Read the model definition and answer for the solid it produces. Units are mm, in the model's axes. A direction names the side the tool comes from. Coordinates: 2 decimals unless noted, no trailing zeros. Loops run counter-clockwise (first coordinate to the right, second up) from the corner with the lowest first, then second, coordinate; pieces in that order, holes last.
Q1. Section D-D (y = 4.55) is taken. Count the separate pieces of the cut face and the enclosed holes in it, then the cut area to 3 significant figures.
Q2. Which of the six approach directions +Z, -Z, +X, -X, +Y, -Y give full straight-line access (tool end or side, diameter ignored) to faces 1 (the face through (166, 3, -151)), 2 (the face through (166, 3, -223)), 3 (the face through (133.805, 3, -141))?
Q3. Section B-B (z = -150.5) is taken. Give the vertices of the cut face in (x, y).
Q4. Flat-ended cylindrical pins translate along their axes: P1, Ø1.8, axis at x = 119.5, y = 2, coming from the +Z side (3 decimals); P2, Ø1, axis at x = 152.5, y = 3, coming from the +Z side; P3, Ø4, axis at x = 126.5, z = -252, coming from the -Y side; P4, Ø3, axis at y = 3, z = -157, coming from the +X side. Find the tip coordinate at first contact, or state that the pin passes through.
Q5. Straight lines are drawn through the part: line 1 (X direction, y = 1.7, z = -183.5); line 2 (Z direction, x = 120, y = 1.45) (3 decimals); line 3 (X direction, y = 3.6, z = -250). For each, find the intervals that lie inside material, in ascending order.
Q6. The mould has two halves that part along X. Classify faces 4 (the face through (146, 3, -144)), 5 (the face through (146, 0, -205)), 6 (the face through (166, 3, -259)): pulls with the +X half, pulls with the -X half, needs draft (parallel to the pull), parting line crosses it, or undercut.
Q7. Section C-C (x = 136.5) is taken. Give the vertices of the cut face in (y, z).
Q8. Section A-A (x = 148.5) is taken. Give the vertices of the cut face in (y, z).
from build123d import *

# Parameters (mm, degrees)
BOSS_EXTRUDE1_DEPTH = 6
SKETCH3_W           = 20
SKETCH3_H           = 20
SKETCH3_W_2         = 5
SKETCH3_H_2         = 10
CUT_EXTRUDE1_DEPTH  = 6


with BuildPart() as part:
    # Sketch2 → Boss-Extrude1 (new body)
    with BuildSketch(Plane(origin=(0, 0, 0), x_dir=(1, 0, 0), z_dir=(0, 1, 0))):
        Polygon((121, 270), (121, 240.585), (115, 240.585), (115, 216.195), (121, 216.195), (121, 191.805), (115, 191.805), (115, 167.415), (121, 167.415), (121, 143.025), (121, 138), (133.805, 138), (133.805, 144), (158.195, 144), (158.195, 138), (171, 138), (171, 167.415), (177, 167.415), (177, 191.805), (171, 191.805), (171, 216.195), (177, 216.195), (177, 240.585), (171, 240.585), (171, 264.975), (171, 270), (158.195, 270), (158.195, 264), (133.805, 264), (133.805, 270), align=None)
    extrude(amount=BOSS_EXTRUDE1_DEPTH)

    # Sketch3 → Cut-Extrude1 (cut)
    with BuildSketch(Plane(origin=(0, 6, 0), x_dir=(1, 0, 0), z_dir=(0, 1, 0))):
        with Locations((151, 244)):
            Rectangle(SKETCH3_W, SKETCH3_H)
        with Locations((168.5, 223)):
            Rectangle(SKETCH3_W_2, SKETCH3_H_2)
        with Locations((168.5, 259)):
            Rectangle(SKETCH3_W_2, SKETCH3_H_2)
        with Locations((168.5, 187)):
            Rectangle(SKETCH3_W_2, SKETCH3_H_2)
        with Locations((168.5, 151)):
            Rectangle(SKETCH3_W_2, SKETCH3_H_2)
    extrude(amount=-CUT_EXTRUDE1_DEPTH, mode=Mode.SUBTRACT)


solid = part.part
Numbers:
1. separate pieces: 1
1. enclosed holes: 2
1. area: 6,290 mm2
2. face 1: +X, +Y, -Y
2. face 2: +Y, -Y
2. face 3: +Z, +Y, -Y
3. outline: (121, 0) - (166, 0) - (166, 6) - (121, 6) - close
4. P1: stops at z = -167.415
4. P2: stops at z = -144
4. P3: stops at y = 0
4. P4: stops at x = 171
5. line 1: x = 115 to 166, 171 to 177
5. line 2: z = -240.585 to -216.195, -191.805 to -167.415
5. line 3: x = 121 to 141, 161 to 171
6. face 4: undercut
6. face 5: needs draft
6. face 6: pulls with the +X half
7. outline: (0, -264) - (6, -264) - (6, -144) - (0, -144) - close
8. outline: (0, -264) - (6, -264) - (6, -254) - (0, -254) - close; (0, -234) - (6, -234) - (6, -144) - (0, -144) - close
